Input: part model. Units: mm. Frame: model coordinates. Face numbers are marked on the shaded views. A direction names the side the tool comes from. Round coordinates to 2 decimals unless told otherwise and drop trailing zeros. Order: outer loops, then holes, each group sorted by start corner. A loop starts at its lowest first (then second) coordinate and runs counter-clockwise, first axis right, second up. Notation, with made-up numbers: M 80,1.25 L 84,1.25 A34 cw 84,36.25 Z; hole C -33,19 d8. An arc over 180 degrees is marked long. One line per question, with ' | ' between items.
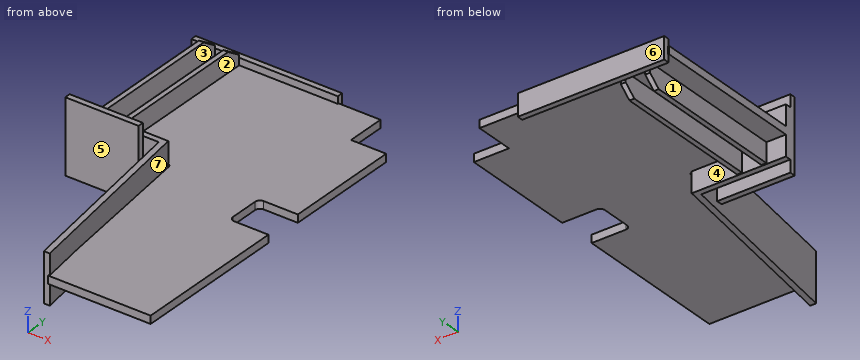
```python
from build123d import *

# Parameters (mm, degrees)
EXTRUDE_1242_DEPTH   = 16
EXTRUDE_2_DEPTH      = 40
EXTRUDE_2_DEPTH_BACK = 56
SKETCH_3_W           = 10
SKETCH_3_H           = 316
CUT_EXTRUDE_1_DEPTH  = 836.425640018
CUT_EXTRUDE_2_DEPTH  = 836.425640018
EXTRUDE_5_DEPTH      = 42
EXTRUDE_5_DEPTH_BACK = 58
EXTRUDE_6_DEPTH      = 14.5
EXTRUDE_6_DEPTH_BACK = 30.5
SKETCH_7_W           = 300
SKETCH_7_H           = 12
SKETCH_8_W           = 150
SKETCH_8_H           = 150
EXTRUDE_7_DEPTH      = 12


with BuildPart() as part:
    # 草图1 → Extrude 1242 (new body)
    with BuildSketch(Plane.XY):
        with BuildLine():
            Line((0, -320), (-70, -320))
            ThreePointArc((-70, -320), (-77.071067812, -322.928932188), (-80, -330))
            Line((-80, -330), (-80, -390))
            ThreePointArc((-80, -390), (-77.071067812, -397.071067812), (-70, -400))
            Line((-70, -400), (0, -400))
            Line((0, -400), (0, -720))
            Line((0, -720), (-210, -720))
            Line((-210, -720), (-259.124034735, -327.007722123))
            ThreePointArc((-259.124034735, -327.007722123), (-261.767837242, -322.002574593), (-267.062257748, -320))
            Line((-267.062257748, -320), (-460, -320))
            Line((-460, -320), (-460, 0))
            Line((-460, 0), (-72, 0))
            Line((-72, 0), (-72, -80))
            Line((-72, -80), (0, -80))
            Line((0, -80), (0, -320))
        make_face()
    extrude(amount=EXTRUDE_1242_DEPTH)

    # 草图3 → 凸台-拉伸2 (add, two sides: drawn at the far end of the back side and taken through both)
    with BuildSketch(Plane.XY.offset(16).offset(-EXTRUDE_2_DEPTH_BACK)):
        with Locations((-415, -160)):
            Rectangle(SKETCH_3_W, SKETCH_3_H)
        with Locations((-365, -160)):
            Rectangle(SKETCH_3_W, SKETCH_3_H)
    extrude(amount=EXTRUDE_2_DEPTH + EXTRUDE_2_DEPTH_BACK)

    # 草图4 → 切除-拉伸1 (cut, through all)
    with BuildSketch(Plane.ZY.offset(420)):
        Polygon((-20, -2), (-45.5, -32), (-45.5, -2), align=None)
    extrude(amount=-CUT_EXTRUDE_1_DEPTH, mode=Mode.SUBTRACT)

    # 草图5 → 切除-拉伸2 (cut, through all)
    with BuildSketch(Plane.ZY.offset(420)):
        Polygon((36, -2), (56, -32), (56, -2), align=None)
    extrude(amount=-CUT_EXTRUDE_2_DEPTH, mode=Mode.SUBTRACT)

    # 草图6 → 凸台-拉伸5 (add, two sides: drawn at the far end of the back side and taken through both)
    with BuildSketch(Plane.XY.offset(16).offset(-EXTRUDE_5_DEPTH_BACK)):
        Polygon((-267.062257748, -318), (-460, -318), (-460, -330), (-277.426505546, -330), (-220.363518026, -718), (-208.234435563, -718), align=None)
    extrude(amount=EXTRUDE_5_DEPTH + EXTRUDE_5_DEPTH_BACK)

    # 草图7 → 凸台-拉伸6 (add, two sides: drawn at the far end of the back side and taken through both)
    with BuildSketch(Plane(origin=(0, 0, 0), x_dir=(-1, 0, 0), z_dir=(0, 0, -1)).offset(-EXTRUDE_6_DEPTH_BACK)):
        with Locations((308, 4)):
            Rectangle(SKETCH_7_W, SKETCH_7_H)
    extrude(amount=EXTRUDE_6_DEPTH + EXTRUDE_6_DEPTH_BACK)

    # 草图8 → 凸台-拉伸7 (add)
    with BuildSketch(Plane.XZ.offset(330)):
        with Locations((-385, 8)):
            Rectangle(SKETCH_8_W, SKETCH_8_H)
    extrude(amount=EXTRUDE_7_DEPTH)


solid = part.part
```
Item 1: Mould query, pull axis Y, two halves, no side actions, for the marked faces 5, 6 and 7. Classes: +Y half, -Y half, draft (parallel to the pull), parting line (faces both ways), or undercut.
Report:
face 5: -Y half | face 6: +Y half | face 7: undercut
Item 2: Section query B-B, the plane y = -39.5. Return loops of the section in (x, z).
Report:
outline: M -460,0 L -420,0 L -420,-40 L -410,-40 L -410,0 L -370,0 L -370,-40 L -360,-40 L -360,0 L -72,0 L -72,16 L -360,16 L -360,56 L -370,56 L -370,16 L -410,16 L -410,56 L -420,56 L -420,16 L -460,16 Z
Item 3: First-contact query: pin 1 (9.5 mm diameter, centred on y = 5.5, z = 6.5, fed in from -X); pin 2 (1 mm diameter, centred on x = -93.5, y = -244.5, fed in from -Z); pin 3 (20 mm diameter, centred on y = -217, z = -10.5, fed in from -X). Flat tips, straight axial feed; report the tip coordinate or a pass-through.
Report:
pin 1: x = -458 | pin 2: z = 0 | pin 3: x = -420
Item 4: Section query D-D, the plane y = -379. Return loops of the section in (x, z) (3 decimals).
Report:
outline: M -270.22,-42 L -258.091,-42 L -258.091,58 L -270.22,58 Z; M -252.625,0 L -80,0 L -80,16 L -252.625,16 Z
Item 5: Section query C-C, the plane z = 45. Return loops of the section in (x, y), plus the area to 3 significant figures.
Report:
outline: M -460,-342 L -310,-342 L -310,-330 L -277.43,-330 L -220.36,-718 L -208.23,-718 L -267.06,-318 L -360,-318 L -360,-15.5 L -370,-15.5 L -370,-318 L -410,-318 L -410,-15.5 L -420,-15.5 L -420,-318 L -460,-318 Z | area: 14,900 mm²
Item 6: Access query for the marked faces 1, 2, 3 and 4. Directions: +Z, -Z, +X, -X, +Y, -Y. A direction counts if a zero-diameter tool reaches every point of the face in a straight line with its end or side. Return the directions, or none.
Report:
face 1: -Z, -X | face 2: +Z, +X | face 3: +Z | face 4: -Z
Item 7: Section query A-A, the plane x = -199. Return loops of the section in (y, z).
Report:
outline: M -720,0 L -2,0 L -2,-14.5 L 10,-14.5 L 10,30.5 L -2,30.5 L -2,16 L -720,16 Z
Item 8: Line query: line 1 along Y through (x, z) = (-296.5, 16.5); line 2 along Z through (x, y) = (-25, -296); line 3 along Y through (x, z) = (-126, 9.5). Output: solid intervals per line, ascending. Write a range as from..to.
Report:
line 1: -330..-318, -2..10 | line 2: 0..16 | line 3: -720..0
